Build history of the part. All positions in model axes, mm. Give positions to 0.01 mm unless a question says otherwise; leave off trailing zeros. Order: outer loops, then holes, each group sorted by start corner. A loop starts at its lowest first (then second) coordinate and runs counter-clockwise, first axis right, second up. Notation, with made-up numbers: (-33, 46) - (8, 46) arc R27 cw to (8, 79) - close; hole circle Ø6 at (61, 81). An arc over 180 degrees is marked (long way). Use a Markdown table: item, result.
from build123d import *

# Parameters (mm, degrees)
BOTTOM_R             = 121
BOTTOM_W             = 10
BOTTOM_H             = 30
BOTTOM_EXTRUDE_DEPTH = 4


with BuildPart() as part:
    # Bottom → Bottom-Extrude (new body)
    with BuildSketch(Plane(origin=(0, 0, 0), x_dir=(-1, 0, 0), z_dir=(0, 1, 0))):
        with Locations(Location((0, 0, 0), (0, 0, 90))):
            Circle(BOTTOM_R)
        with Locations((100, 0)):
            Rectangle(BOTTOM_W, BOTTOM_H, mode=Mode.SUBTRACT)
        with Locations((-100, 0)):
            Rectangle(BOTTOM_W, BOTTOM_H, mode=Mode.SUBTRACT)
    extrude(amount=BOTTOM_EXTRUDE_DEPTH)


solid = part.part
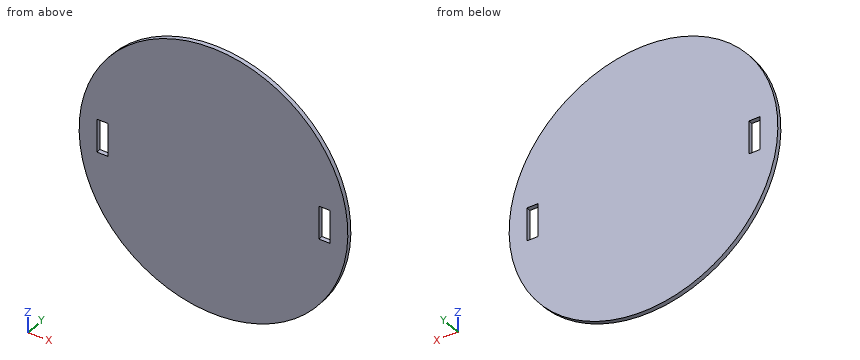
1) Wall check: line 1 (Z direction, x = -2.5, y = 2.95); line 2 (X direction, y = 1.1, z = -8); line 3 (Z direction, x = 61, y = 1.5). Give the ranges that are in metal, low to high. Write a range as from..to.
Computed:
| item | result |
|---|---|
| line 1 | z = -120.97..120.97 |
| line 2 | x = -120.74..-105, -95..95, 105..120.74 |
| line 3 | z = -104.5..104.5 |
2) Slice it at A-A (z = 0). Write the cut outline in (x, y).
Computed:
| item | result |
|---|---|
| outline | (-121, 0) - (-105, 0) - (-105, 4) - (-121, 4) - close; (-95, 0) - (95, 0) - (95, 4) - (-95, 4) - close; (105, 0) - (121, 0) - (121, 4) - (105, 4) - close |
3) Pin check, flat tips, straight feed: P1, Ø2, axis at y = 2, z = 4, coming from the -X side; P2, Ø1.2, axis at x = 102, y = 2.5, coming from the +Z side; P3, Ø2, axis at x = -98.5, y = 2.5, coming from the +Z side. Stop position of each tip, or through.
Computed:
| item | result |
|---|---|
| P1 | stops at x = -120.96 |
| P2 | stops at z = 66.02 |
| P3 | stops at z = 71.66 |
4) Slice it at D-D (z = 104). Write the cut outline in (x, y), and give its area (3 significant figures).
Computed:
| item | result |
|---|---|
| outline | (-61.85, 0) - (61.85, 0) - (61.85, 4) - (-61.85, 4) - close |
| area | 495 mm² |
5) Slice it at B-B (y = 0.7). Write the cut outline in (x, z), and give its area (3 significant figures).
Computed:
| item | result |
|---|---|
| outline | circle Ø242 at (0, 0); hole (-105, -15) - (-95, -15) - (-95, 15) - (-105, 15) - close; hole (95, -15) - (105, -15) - (105, 15) - (95, 15) - close |
| area | 45,400 mm² |
6) Slice it at C-C (x = 39.5). Write the cut outline in (y, z), and give its area (3 significant figures).
Computed:
| item | result |
|---|---|
| outline | (0, -114.37) - (4, -114.37) - (4, 114.37) - (0, 114.37) - close |
| area | 915 mm² |
